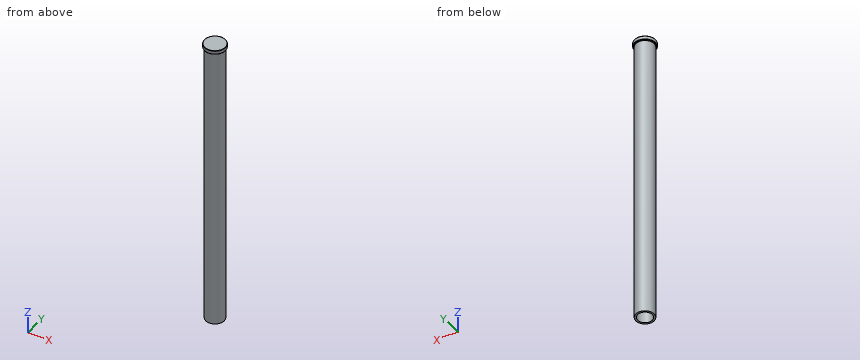
from build123d import *

# Parameters (mm, degrees)
SKETCH1_R           = 9
BOSS_EXTRUDE1_DEPTH = 80
SKETCH2_R           = 2
CUT_EXTRUDE1_DEPTH  = 15
SKETCH3_R           = 9
SKETCH3_R_2         = 2.5
CUT_EXTRUDE3_DEPTH  = 112
SKETCH6_R           = 2.86034934
BOSS_EXTRUDE2_DEPTH = 1
FILLET1_R           = 0.1


with BuildPart() as part:
    # Sketch1 → Boss-Extrude1 (new body)
    with BuildSketch(Plane.XY):
        Circle(SKETCH1_R)
    extrude(amount=BOSS_EXTRUDE1_DEPTH)

    # Sketch2 → Cut-Extrude1 (cut)
    with BuildSketch(Plane(origin=(0, 0, 0), x_dir=(-1, 0, 0), z_dir=(0, 0, -1))):
        Circle(SKETCH2_R)
    extrude(amount=-CUT_EXTRUDE1_DEPTH, mode=Mode.SUBTRACT)

    # Sketch3 → Cut-Extrude3 (cut)
    with BuildSketch(Plane(origin=(0, 0, 0), x_dir=(-1, 0, 0), z_dir=(0, 0, -1))):
        Circle(SKETCH3_R)
        Circle(SKETCH3_R_2, mode=Mode.SUBTRACT)
    extrude(amount=-CUT_EXTRUDE3_DEPTH, mode=Mode.SUBTRACT)

    # Sketch6 → Boss-Extrude2 (add)
    with BuildSketch(Plane.XY.offset(80)):
        Circle(SKETCH6_R)
    extrude(amount=-BOSS_EXTRUDE2_DEPTH)

    # Fillet1
    fillet1_edges = [part.edges().sort_by_distance(p)[0] for p in [
        (2.5, 0, 79),
        (-2.86034934, 0, 79),
        (-2.86034934, 0, 80),
    ]]
    fillet(fillet1_edges, radius=FILLET1_R)


solid = part.part
Geometry: final body of the model. Coordinates: model frame, mm. Give positions to 0.01 mm unless a question says otherwise; leave off trailing zeros. Loops run counter-clockwise (first coordinate to the right, second up) from the corner with the lowest first, then second, coordinate; pieces in that order, holes last. Notation, with made-up numbers: (-4, 53.5) - (23, 53.5) arc R13 cw to (23, 64.5) - close; hole circle Ø5 at (75.25, -20). An arc over 180 degrees is marked (long way). One line per question, with ' | ' between items. Start each with the question number.
(1) Contact query for flat-ended pins moving along their axis: pin 1 (1.5 mm diameter, centred on x = 1, z = 16.5, fed in from -Y); pin 2 (1.5 mm diameter, centred on y = 1.5, z = 50, fed in from -X); pin 3 (3 mm diameter, centred on x = 0, y = 0, fed in from -Z). Output: stop coordinate, or through.
(2) Ray query, line 1 (Y direction, x = 0, z = 8.5); line 2 (Z direction, x = 0.25, y = 0.4); line 3 (X direction, y = -0.2, z = 44). Return the intervals inside material, ascending. Write a range as from..to.
(3) Section query C-C on z = 20.5. Return loops of the section in (x, y).
(4) Section query A-A on y = 0. Return loops of the section in (x, z), then the cut area to 3 significant figures.
The answers:
1) pin 1: y = -2.49 | pin 2: x = -2.38 | pin 3: z = 15
2) line 1: -2.5..-2, 2..2.5 | line 2: 15..80 | line 3: -2.49..2.49
3) outline: circle Ø5 at (0, 0)
4) outline: (-2.86, 79.1) arc R0.1 ccw to (-2.76, 79) - (-2.6, 79) arc R0.1 cw to (-2.5, 78.9) - (-2.5, 0) - (-2, 0) - (-2, 15) - (2, 15) - (2, 0) - (2.5, 0) - (2.5, 78.9) arc R0.1 cw to (2.6, 79) - (2.76, 79) arc R0.1 ccw to (2.86, 79.1) - (2.86, 79.9) arc R0.1 ccw to (2.76, 80) - (-2.76, 80) arc R0.1 ccw to (-2.86, 79.9) - close | area: 341 mm2
